Geometry: see drawing. Coordinates: mm, zero at the bounding-box minimum. Give positions to 0.01 mm unless a question says otherwise; leave off trailing zeros. Write each loop counter-clockwise with the first axis right and the second up, starting at its lowest first coordinate (ties: lowest second). Pieces come first, ordered by that corner, then holes. Notation, with made-up numbers: (12.5, -9) - (66.5, -9) arc R12 ccw to (66.5, 2) - close; hole circle Ø10 at (30, -22.5). An arc over 180 degrees is marked (long way). Return JSON: item names as keys, results as strings.
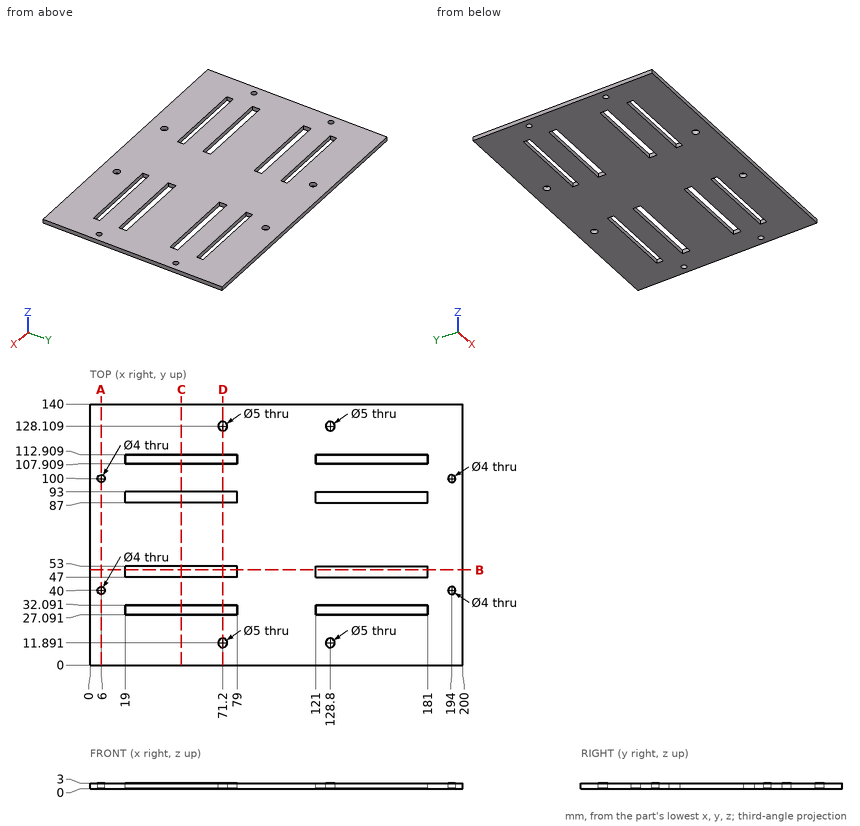
Q1. Section query A-A, the plane x = 6. Return the cut outline in (y, z).
Answer key:
{"outline": "(0, 0) - (38, 0) - (38, 3) - (0, 3) - close; (42, 0) - (98, 0) - (98, 3) - (42, 3) - close; (102, 0) - (140, 0) - (140, 3) - (102, 3) - close"}
Q2. Section query B-B, the plane y = 51. Return the cut outline in (x, z), plus the area to 3 significant figures.
Answer key:
{"outline": "(0, 0) - (19, 0) - (19, 3) - (0, 3) - close; (79, 0) - (121, 0) - (121, 3) - (79, 3) - close; (181, 0) - (200, 0) - (200, 3) - (181, 3) - close", "area": "240 mm^2"}
Q3. Section query D-D, the plane x = 71.2. Return the cut outline in (y, z), plus the area to 3 significant figures.
Answer key:
{"outline": "(0, 0) - (9.39, 0) - (9.39, 3) - (0, 3) - close; (14.39, 0) - (27.09, 0) - (27.09, 3) - (14.39, 3) - close; (32.09, 0) - (47, 0) - (47, 3) - (32.09, 3) - close; (53, 0) - (87, 0) - (87, 3) - (53, 3) - close; (93, 0) - (107.91, 0) - (107.91, 3) - (93, 3) - close; (112.91, 0) - (125.61, 0) - (125.61, 3) - (112.91, 3) - close; (130.61, 0) - (140, 0) - (140, 3) - (130.61, 3) - close", "area": "324 mm^2"}
Q4. Section query C-C, the plane x = 49. Return the cut outline in (y, z).
Answer key:
{"outline": "(0, 0) - (27.09, 0) - (27.09, 3) - (0, 3) - close; (32.09, 0) - (47, 0) - (47, 3) - (32.09, 3) - close; (53, 0) - (87, 0) - (87, 3) - (53, 3) - close; (93, 0) - (107.91, 0) - (107.91, 3) - (93, 3) - close; (112.91, 0) - (140, 0) - (140, 3) - (112.91, 3) - close"}
Q5. Material intervals for probe 1 along Y at (x, z) = (6, 1.25); probe 2 along Y at (x, z) = (28, 2.6); probe 3 along X at (y, z) = (48.5, 1.9), sorted ascending. Write a range as [from, to].
Answer key:
{"probe 1": "y = [0, 38], [42, 98], [102, 140]", "probe 2": "y = [0, 27.09], [32.09, 47], [53, 87], [93, 107.91], [112.91, 140]", "probe 3": "x = [0, 19], [79, 121], [181, 200]"}
